Geometry check sheet. Reference: the model listing, model coordinates, mm. A direction names the side the tool comes from. Give positions to 0.01 mm unless a question says otherwise; leave off trailing zeros. Loops run counter-clockwise (first coordinate to the right, second up) from the corner with the lowest first, then second, coordinate; pieces in that order, holes last. Notation, with made-up numbers: (76, 56.25) -> (114, 56.25) arc R23 ccw to (114, 86.25) -> close; hole circle Ø7 at (6.25, 81). An arc over 180 degrees is marked (long way). Answer as a JSON object with one key per item and string values.
from build123d import *

# Parameters (mm, degrees)
SKETCH_1_W          = 38
SKETCH_1_H          = 75
EXTRUDE_1_DEPTH     = 30.73
SKETCH_2_R          = 10
EXTRUDE_2_DEPTH     = 7.11
SKETCH_3_W          = 30.7
SKETCH_3_H          = 10.4
EXTRUDE_3_DEPTH     = 6.4
SKETCH_5_W          = 30.5
SKETCH_5_H          = 67
CUT_EXTRUDE_1_DEPTH = 60.609353293
CUT_EXTRUDE_2_REACH = 87.153
SKETCH_6_W          = 9.8
SKETCH_6_H          = 20.33
CUT_EXTRUDE_3_REACH = 69.753
SKETCH_8_R          = 1.4
CUT_EXTRUDE_4_DEPTH = 7.4
SKETCH_10_W         = 6
SKETCH_10_H         = 30.73
CUT_EXTRUDE_5_DEPTH = 1.5


with BuildPart() as part:
    # 草图1 → 凸台-拉伸1 (new body)
    with BuildSketch(Plane(origin=(0, 0, 0), x_dir=(1, 0, 0), z_dir=(0, 1, 0))):
        Rectangle(SKETCH_1_W, SKETCH_1_H)
    extrude(amount=EXTRUDE_1_DEPTH)

    # 草图2 → 凸台-拉伸2 (add)
    with BuildSketch(Plane.ZY.offset(19)):
        with Locations(Location((-18.89, 13.38, 0), (0, 0, 180))):
            Circle(SKETCH_2_R)
    extrude_2 = extrude(amount=EXTRUDE_2_DEPTH)

    # 草图3 → 凸台-拉伸3 (add)
    with BuildSketch(Plane(origin=(0, 0, -37.5), x_dir=(-1, 0, 0), z_dir=(0, 0, -1))):
        with Locations((0, 25.53)):
            Rectangle(SKETCH_3_W, SKETCH_3_H)
    extrude_3 = extrude(amount=EXTRUDE_3_DEPTH)

    # 草图5 → 切除-拉伸1 (cut, through all)
    with BuildSketch(Plane(origin=(0, 30.73, 0), x_dir=(1, 0, 0), z_dir=(0, 1, 0))):
        Rectangle(SKETCH_5_W, SKETCH_5_H)
    extrude(amount=-CUT_EXTRUDE_1_DEPTH, mode=Mode.SUBTRACT)

    # 镜向2: 凸台-拉伸2 across plane
    add(extrude_2.mirror(Plane(origin=(0, 0, 0), x_dir=(0, 0, 1), z_dir=(1, 0, 0))))

    # 草图6 → 切除-拉伸2 (cut, up to next)
    with BuildSketch(Plane(origin=(0, 0, -37.5), x_dir=(-1, 0, 0), z_dir=(0, 0, -1)), mode=Mode.PRIVATE) as cut_extrude_2_sk1:
        with Locations((0, 10.165)):
            Rectangle(SKETCH_6_W, SKETCH_6_H)
    cut_extrude_2_tool1 = extrude(cut_extrude_2_sk1.sketch, amount=-CUT_EXTRUDE_2_REACH, mode=Mode.PRIVATE) & part.part
    add(cut_extrude_2_tool1.solids().sort_by_distance((0, 10.165, -37.5))[0], mode=Mode.SUBTRACT)

    # 草图7 → 切除-拉伸3 (cut, up to next)
    with BuildSketch(Plane(origin=(15.35, 0, 0), x_dir=(0, 0, -1), z_dir=(1, 0, 0)), mode=Mode.PRIVATE) as cut_extrude_3_sk1:
        Polygon((37.5, 20.33), (43.9, 25.33022801), (43.9, 20.33), align=None)
    cut_extrude_3_tool1 = extrude(cut_extrude_3_sk1.sketch, amount=-CUT_EXTRUDE_3_REACH, mode=Mode.PRIVATE) & part.part
    cut_extrude_3 = cut_extrude_3_tool1.solids().sort_by_distance((15.35, 21.996743, -41.766667))[0]
    add(cut_extrude_3, mode=Mode.SUBTRACT)

    # 镜向4: 凸台-拉伸3, 切除-拉伸3 across plane
    add(extrude_3.mirror(Plane.XY))
    add(cut_extrude_3.mirror(Plane.XY), mode=Mode.SUBTRACT)

    # 草图8 → 切除-拉伸4 (cut)
    with BuildSketch(Plane(origin=(0, 30.73, 0), x_dir=(1, 0, 0), z_dir=(0, 1, 0))):
        with Locations(Location((-8.5, 37.5, 0), (0, 0, 270))):
            Circle(SKETCH_8_R)
        with Locations(Location((8.5, 37.5, 0), (0, 0, 90))):
            Circle(SKETCH_8_R)
        with Locations(Location((8.5, -37.5, 0), (0, 0, 270))):
            Circle(SKETCH_8_R)
        with Locations(Location((-8.5, -37.5, 0), (0, 0, 90))):
            Circle(SKETCH_8_R)
    extrude(amount=-CUT_EXTRUDE_4_DEPTH, mode=Mode.SUBTRACT)

    # 草图10 → 切除-拉伸5 (cut)
    with BuildSketch(Plane(origin=(-15.25, 0, 0), x_dir=(0, 0, -1), z_dir=(1, 0, 0))):
        with Locations((11, 15.365)):
            Rectangle(SKETCH_10_W, SKETCH_10_H)
    extrude(amount=-CUT_EXTRUDE_5_DEPTH, mode=Mode.SUBTRACT)


solid = part.part
1) Section check D-D on y = 28. Record the cut outline in (x, z), plus the area to 3 significant figures.
Geometry check:
{"outline": "(-19, -37.5) -> (-15.35, -37.5) -> (-15.35, -43.9) -> (15.35, -43.9) -> (15.35, -37.5) -> (19, -37.5) -> (19, 37.5) -> (15.35, 37.5) -> (15.35, 43.9) -> (-15.35, 43.9) -> (-15.35, 37.5) -> (-19, 37.5) -> close; hole (-16.75, -14) -> (-15.25, -14) -> (-15.25, -33.5) -> (15.25, -33.5) -> (15.25, 33.5) -> (-15.25, 33.5) -> (-15.25, -8) -> (-16.75, -8) -> close; hole circle Ø2.8 at (-8.5, -37.5); hole circle Ø2.8 at (-8.5, 37.5); hole circle Ø2.8 at (8.5, -37.5); hole circle Ø2.8 at (8.5, 37.5)", "area": "1,170 mm2"}
2) Depth check by flat-ended pin: P1, Ø4.5, axis at y = 13.5, z = -34.5, coming from the -X side; P2, Ø1.9, axis at y = 26, z = -40, coming from the +X side; P3, Ø5, axis at y = 26, z = 41, coming from the -X side. Enter the tip coordinate at first touch or a pass-through.
Geometry check:
{"P1": "stops at x = -19", "P2": "stops at x = 15.35", "P3": "stops at x = -15.35"}
3) Section check C-C on y = 13.38. Record the cut outline in (x, z).
Geometry check:
{"outline": "(-26.11, -28.89) -> (-19, -28.89) -> (-19, -37.5) -> (-4.9, -37.5) -> (-4.9, -33.5) -> (-15.25, -33.5) -> (-15.25, -14) -> (-16.75, -14) -> (-16.75, -8) -> (-15.25, -8) -> (-15.25, 33.5) -> (15.25, 33.5) -> (15.25, -33.5) -> (4.9, -33.5) -> (4.9, -37.5) -> (19, -37.5) -> (19, -28.89) -> (26.11, -28.89) -> (26.11, -8.89) -> (19, -8.89) -> (19, 37.5) -> (-19, 37.5) -> (-19, -8.89) -> (-26.11, -8.89) -> close"}
4) Section check B-B on x = -12.5. Record the cut outline in (y, z).
Geometry check:
{"outline": "(0, -37.5) -> (20.33, -37.5) -> (25.33, -43.9) -> (30.73, -43.9) -> (30.73, -33.5) -> (0, -33.5) -> close; (0, 33.5) -> (30.73, 33.5) -> (30.73, 43.9) -> (25.33, 43.9) -> (20.33, 37.5) -> (0, 37.5) -> close"}
5) Draft check along Z on faces 4 (the face through (0, 28, 43.9)), 5 (the face through (9, 23.33, 37)), 6 (the face through (19, 15, 1)). Enter one of: pulls with the +Z half, pulls with the -Z half, needs draft (parallel to the pull), parting line crosses it, or undercut.
Geometry check:
{"face 4": "pulls with the +Z half", "face 5": "undercut", "face 6": "needs draft"}
6) Tool access check on faces 1 (the face through (15.35, 27, 41)), 2 (the face through (0, 20.33, -35)), 3 (the face through (-8, 23.33, -38)). Record the directions out of +Z, -Z, +X, -X, +Y, -Y that give a thin tool (end or side, any length) a straight path to the whole face; none if there is none.
Geometry check:
{"face 1": "+Z, +X, +Y, -Y", "face 2": "-Z, -Y", "face 3": "+Y"}
7) Section check A-A on z = -18.89. Record the cut outline in (x, y), plus the area to 3 significant figures.
Geometry check:
{"outline": "(-26.11, 3.38) -> (-19, 3.38) -> (-19, 0) -> (-15.25, 0) -> (-15.25, 30.73) -> (-19, 30.73) -> (-19, 23.38) -> (-26.11, 23.38) -> close; (15.25, 0) -> (19, 0) -> (19, 3.38) -> (26.11, 3.38) -> (26.11, 23.38) -> (19, 23.38) -> (19, 30.73) -> (15.25, 30.73) -> close", "area": "515 mm2"}
8) Material ranges on line 1 along X through (y, z) = (26.5, 25.5); line 2 along X through (y, z) = (26, 37); line 3 along Z through (x, y) = (-16, 9), recorded low to high. Write a range as from..to.
Geometry check:
{"line 1": "x = -19..-15.25, 15.25..19", "line 2": "x = -19..-9.81, -7.19..7.19, 9.81..19", "line 3": "z = -37.5..-14, -8..37.5"}
